Here's how the part is built. I have some questions about the finished solid (model axes, mm). A direction names the side the tool comes from. Coordinates: 2 decimals unless noted, no trailing zeros. Write each loop counter-clockwise with the first axis right and the second up, starting at its lowest first coordinate (ties: lowest second). Pieces come first, ordered by that corner, then holes.
Item 1: I want a section at A-A (x = 0). Please give me the cut outline in (y, z) (3 decimals).
Item 2: I'm going to push flat-ended pins straight in: P1, Ø3, axis at y = 1, z = -22, coming from the +X side; P2, Ø4, axis at y = -3, z = -37, coming from the -X side; P3, Ø2, axis at x = -3, z = -39, coming from the +Y side. Where does each tip first touch, or does it pass through?
Item 3: For faces 1 (the face through (2, 2, 0)), 2 (the face through (-2, -1, 4.826)), 3 (the face through (1.727, -0.978, 3.261)), which set-ups out of +Z, -Z, +X, -X, +Y, -Y let a thin tool reach every point of the face, with its end or its side?
Item 4: If we mould it in two halves opening along Y, with no side actions, what happens to faces 4 (the face through (-0.52, -3.93, 2.13)), 5 (the face through (0, 0, -44.45)), 6 (the face through (0, 1.984, 3))? For each: pulls with the +Y half, pulls with the -Y half, needs draft (parallel to the pull), parting line crosses it, or undercut.
Item 5: Please list where these lines run through material, in increasing order: line 1 (Y direction, x = -0.75, z = -37); line 2 (Z direction, x = 2.5, y = 0.75); line 3 (Z direction, x = -0.75, y = 0.25).
Item 6: I want a section at B-B (z = -33). Please give me the cut outline in (x, y).
Autodesk Inventor part; units mm, degrees
ref_plane "YZ Plane" through (0, 0, 0) normal (1, 0, 0) x (0, 1, 0)
ref_plane "XZ Plane" through (0, 0, 0) normal (0, 1, 0) x (-1, 0, 0)
ref_plane "XY Plane" through (0, 0, 0) normal (0, 0, 1) x (1, 0, 0)
sketch "Sketch1" plane through (0, 0, 0) normal (0, 0, 1) x (1, 0, 0)
  circle A0 centre (0, 0) radius 3.9624
  dimension "d0" = 7.9248
extrude "Extrusion1" add sketch "Sketch1" along normal blind 4.826
sketch "Sketch2" plane through (0, 0, 0) normal (0, 0, -1) x (-1, 0, 0)
  circle A0 centre (0, 0) radius 3.9624
  circle A1 centre (0, 0) radius 2.413
  dimension "d3" = 4.826
extrude "Extrusion2" add sketch "Sketch2" along normal blind 44.45 contours A1
sketch "Sketch3" plane through (0, 0, 4.826) normal (0, 0, 1) x (1, 0, 0)
  circle A0 centre (0, 0) radius 3.9624
  line L0 (-1.1457, 1.9844) -> (1.1457, 1.9844)
  line L1 (1.1457, 1.9844) -> (2.2914, 0)
  line L2 (2.2914, 0) -> (1.1457, -1.9844)
  line L3 (1.1457, -1.9844) -> (-1.1457, -1.9844)
  line L4 (-1.1457, -1.9844) -> (-2.2914, 0)
  line L5 (-2.2914, 0) -> (-1.1457, 1.9844)
  dimension "d6" = 3.9688
extrude "Extrusion3" cut sketch "Sketch3" against normal blind 3.175 contours L0 L1 L2 L3 L4 L5
thread "Thread1"
chamfer "Chamfer1" distance 0.508 angle 45 1 edges at (2.413, 0, -44.45)
chamfer "Chamfer2" distance 0.508 angle 45 1 edges at (-3.9624, 0, 4.826)
properties part number "10-32 x1000" material "Steel"
Answer:
1. outline: (-3.962, 0) - (-2.413, 0) - (-2.413, -43.942) - (-1.905, -44.45) - (1.905, -44.45) - (2.413, -43.942) - (2.413, 0) - (3.962, 0) - (3.962, 4.318) - (3.454, 4.826) - (1.984, 4.826) - (1.984, 1.651) - (-1.984, 1.651) - (-1.984, 4.826) - (-3.454, 4.826) - (-3.962, 4.318) - close
2. P1: stops at x = 2.41
2. P2: stops at x = -2.2
2. P3: stops at y = 1.35
3. face 1: -Z
3. face 2: +Z, +X, -X, +Y, -Y
3. face 3: +Z
4. face 4: parting line crosses it
4. face 5: needs draft
4. face 6: undercut
5. line 1: y = -2.29 to 2.29
5. line 2: z = 0 to 4.83
5. line 3: z = -44.45 to 1.65
6. outline: circle Ø4.83 at (0, 0)
